```python
from build123d import *

# Parameters (mm, degrees)
SKETCH1_W                            = 609.6
SKETCH1_H                            = 609.6
LEXAN_BOSS_EXTRUDE1_DEPTH            = 12.7
HOUSING_NEST_HOLE_CUT_EXTRUDE1_REACH = 14.7
SKETCH5_W                            = 280
SKETCH5_H                            = 170
CUT_EXTRUDE7_REACH                   = 14.7
SKETCH6_R                            = 3.25
SKETCH9_R                            = 3.25
CUT_EXTRUDE6_DEPTH                   = 13.7
LPATTERN5_COUNT                      = 5
LPATTERN5_PITCH                      = 20
LPATTERN5_COL_COUNT                  = 5
LPATTERN5_COL_PITCH                  = 20
FILLET3_R                            = 10


with BuildPart() as part:
    # Sketch1 → Lexan Boss-Extrude1 (new body)
    with BuildSketch(Plane(origin=(0, 0, 0), x_dir=(1, 0, 0), z_dir=(0, 1, 0))):
        Rectangle(SKETCH1_W, SKETCH1_H)
    extrude(amount=LEXAN_BOSS_EXTRUDE1_DEPTH)

    # Sketch5 → Housing nest hole Cut-Extrude1 (cut, up to next)
    with BuildSketch(Plane.XZ, mode=Mode.PRIVATE) as housing_nest_hole_cut_extrude1_sk1:
        Rectangle(SKETCH5_W, SKETCH5_H)
    housing_nest_hole_cut_extrude1_tool1 = extrude(housing_nest_hole_cut_extrude1_sk1.sketch, amount=-HOUSING_NEST_HOLE_CUT_EXTRUDE1_REACH, mode=Mode.PRIVATE) & part.part
    add(housing_nest_hole_cut_extrude1_tool1.solids().sort_by_distance((0, 0, 0))[0], mode=Mode.SUBTRACT)

    # Sketch6 → Cut-Extrude7 (cut, up to next)
    with BuildSketch(Plane.XZ, mode=Mode.PRIVATE) as cut_extrude7_sk1:
        with Locations((-284.8, 275)):
            Circle(SKETCH6_R)
    cut_extrude7_tool1 = extrude(cut_extrude7_sk1.sketch, amount=-CUT_EXTRUDE7_REACH, mode=Mode.PRIVATE) & part.part
    add(cut_extrude7_tool1.solids().sort_by_distance((-284.8, 0, 275))[0], mode=Mode.SUBTRACT)
    # Sketch6 → Cut-Extrude7 (cut, up to next)
    with BuildSketch(Plane.XZ, mode=Mode.PRIVATE) as cut_extrude7_sk2:
        with Locations((-284.8, 0)):
            Circle(SKETCH6_R)
    cut_extrude7_tool2 = extrude(cut_extrude7_sk2.sketch, amount=-CUT_EXTRUDE7_REACH, mode=Mode.PRIVATE) & part.part
    add(cut_extrude7_tool2.solids().sort_by_distance((-284.8, 0, 0))[0], mode=Mode.SUBTRACT)
    # Sketch6 → Cut-Extrude7 (cut, up to next)
    with BuildSketch(Plane.XZ, mode=Mode.PRIVATE) as cut_extrude7_sk3:
        with Locations((-284.8, -275)):
            Circle(SKETCH6_R)
    cut_extrude7_tool3 = extrude(cut_extrude7_sk3.sketch, amount=-CUT_EXTRUDE7_REACH, mode=Mode.PRIVATE) & part.part
    add(cut_extrude7_tool3.solids().sort_by_distance((-284.8, 0, -275))[0], mode=Mode.SUBTRACT)
    # Sketch6 → Cut-Extrude7 (cut, up to next)
    with BuildSketch(Plane.XZ, mode=Mode.PRIVATE) as cut_extrude7_sk4:
        with Locations((284.8, -275)):
            Circle(SKETCH6_R)
    cut_extrude7_tool4 = extrude(cut_extrude7_sk4.sketch, amount=-CUT_EXTRUDE7_REACH, mode=Mode.PRIVATE) & part.part
    add(cut_extrude7_tool4.solids().sort_by_distance((284.8, 0, -275))[0], mode=Mode.SUBTRACT)
    # Sketch6 → Cut-Extrude7 (cut, up to next)
    with BuildSketch(Plane.XZ, mode=Mode.PRIVATE) as cut_extrude7_sk5:
        with Locations((284.8, 0)):
            Circle(SKETCH6_R)
    cut_extrude7_tool5 = extrude(cut_extrude7_sk5.sketch, amount=-CUT_EXTRUDE7_REACH, mode=Mode.PRIVATE) & part.part
    add(cut_extrude7_tool5.solids().sort_by_distance((284.8, 0, 0))[0], mode=Mode.SUBTRACT)
    # Sketch6 → Cut-Extrude7 (cut, up to next)
    with BuildSketch(Plane.XZ, mode=Mode.PRIVATE) as cut_extrude7_sk6:
        with Locations((284.8, 275)):
            Circle(SKETCH6_R)
    cut_extrude7_tool6 = extrude(cut_extrude7_sk6.sketch, amount=-CUT_EXTRUDE7_REACH, mode=Mode.PRIVATE) & part.part
    add(cut_extrude7_tool6.solids().sort_by_distance((284.8, 0, 275))[0], mode=Mode.SUBTRACT)
    # Sketch6 → Cut-Extrude7 (cut, up to next)
    with BuildSketch(Plane.XZ, mode=Mode.PRIVATE) as cut_extrude7_sk7:
        with Locations((-225, 284.8)):
            Circle(SKETCH6_R)
    cut_extrude7_tool7 = extrude(cut_extrude7_sk7.sketch, amount=-CUT_EXTRUDE7_REACH, mode=Mode.PRIVATE) & part.part
    add(cut_extrude7_tool7.solids().sort_by_distance((-225, 0, 284.8))[0], mode=Mode.SUBTRACT)
    # Sketch6 → Cut-Extrude7 (cut, up to next)
    with BuildSketch(Plane.XZ, mode=Mode.PRIVATE) as cut_extrude7_sk8:
        with Locations((0, 284.8)):
            Circle(SKETCH6_R)
    cut_extrude7_tool8 = extrude(cut_extrude7_sk8.sketch, amount=-CUT_EXTRUDE7_REACH, mode=Mode.PRIVATE) & part.part
    add(cut_extrude7_tool8.solids().sort_by_distance((0, 0, 284.8))[0], mode=Mode.SUBTRACT)
    # Sketch6 → Cut-Extrude7 (cut, up to next)
    with BuildSketch(Plane.XZ, mode=Mode.PRIVATE) as cut_extrude7_sk9:
        with Locations((225, 284.8)):
            Circle(SKETCH6_R)
    cut_extrude7_tool9 = extrude(cut_extrude7_sk9.sketch, amount=-CUT_EXTRUDE7_REACH, mode=Mode.PRIVATE) & part.part
    add(cut_extrude7_tool9.solids().sort_by_distance((225, 0, 284.8))[0], mode=Mode.SUBTRACT)
    # Sketch6 → Cut-Extrude7 (cut, up to next)
    with BuildSketch(Plane.XZ, mode=Mode.PRIVATE) as cut_extrude7_sk10:
        with Locations((225, -284.8)):
            Circle(SKETCH6_R)
    cut_extrude7_tool10 = extrude(cut_extrude7_sk10.sketch, amount=-CUT_EXTRUDE7_REACH, mode=Mode.PRIVATE) & part.part
    add(cut_extrude7_tool10.solids().sort_by_distance((225, 0, -284.8))[0], mode=Mode.SUBTRACT)
    # Sketch6 → Cut-Extrude7 (cut, up to next)
    with BuildSketch(Plane.XZ, mode=Mode.PRIVATE) as cut_extrude7_sk11:
        with Locations((0, -284.8)):
            Circle(SKETCH6_R)
    cut_extrude7_tool11 = extrude(cut_extrude7_sk11.sketch, amount=-CUT_EXTRUDE7_REACH, mode=Mode.PRIVATE) & part.part
    add(cut_extrude7_tool11.solids().sort_by_distance((0, 0, -284.8))[0], mode=Mode.SUBTRACT)
    # Sketch6 → Cut-Extrude7 (cut, up to next)
    with BuildSketch(Plane.XZ, mode=Mode.PRIVATE) as cut_extrude7_sk12:
        with Locations((-225, -284.8)):
            Circle(SKETCH6_R)
    cut_extrude7_tool12 = extrude(cut_extrude7_sk12.sketch, amount=-CUT_EXTRUDE7_REACH, mode=Mode.PRIVATE) & part.part
    add(cut_extrude7_tool12.solids().sort_by_distance((-225, 0, -284.8))[0], mode=Mode.SUBTRACT)

    # Sketch9 → Cut-Extrude6 (cut, through all)
    with BuildSketch(Plane(origin=(0, 12.7, 0), x_dir=(1, 0, 0), z_dir=(0, 1, 0))):
        with Locations((-180, 0)):
            Circle(SKETCH9_R)
        with Locations((180, 0)):
            Circle(SKETCH9_R)
    cut_extrude6 = extrude(amount=-CUT_EXTRUDE6_DEPTH, mode=Mode.SUBTRACT)

    # LPattern5: Cut-Extrude6 ×5
    with Locations(*[(0, 0, i * LPATTERN5_PITCH) for i in range(1, LPATTERN5_COUNT)]):
        add(cut_extrude6, mode=Mode.SUBTRACT)

    # LPattern5 col: Cut-Extrude6 ×5
    with Locations(*[(0, 0, -i * LPATTERN5_COL_PITCH) for i in range(1, LPATTERN5_COL_COUNT)]):
        add(cut_extrude6, mode=Mode.SUBTRACT)

    # Fillet3
    fillet3_edges = [part.edges().sort_by_distance(p)[0] for p in [
        (304.8, 6.35, 304.8),
        (-304.8, 6.35, 304.8),
        (-304.8, 6.35, -304.8),
        (304.8, 6.35, -304.8),
    ]]
    fillet(fillet3_edges, radius=FILLET3_R)


solid = part.part
```
Design review of the part built by this model. Coordinates are the model's own, in mm. Give positions to 0.01 mm unless a question says otherwise; leave off trailing zeros. Return JSON: item names as keys, results as strings. Group by question number.
(1) We need section A-A, the plane y = 8.5. Give the number of separate pieces and of enclosed holes in the cut face, then the cut area to 3 significant figures.
(2) To check wall thickness, follow probe 1 along Z at (x, y) = (-225, 8.75); probe 2 along X at (y, z) = (9.25, 40); probe 3 along Z at (x, y) = (284.8, 2.75). State the ranges of each line that lie inside material, in increasing order.
(3) Insertion check: pin 1 (5 mm diameter, centred on x = 0, z = -284.8, fed in from +Y). The pin has a flat end and moves straight along its axis. Give the tip position at first contact, or say it passes through.
Reported:
{
 "1": {"separate pieces": "1", "enclosed holes": "31", "area": "323,000 mm2"},
 "2": {"probe 1": "z = -304.8 to -288.05, -281.55 to 281.55, 288.05 to 304.8", "probe 2": "x = -304.8 to -183.25, -176.75 to -140, 140 to 176.75, 183.25 to 304.8", "probe 3": "z = -304.8 to -278.25, -271.75 to -3.25, 3.25 to 271.75, 278.25 to 304.8"},
 "3": {"pin 1": "passes through"}
}
